For this review, take the finished solid that the model builds, in its own axes (mm). A direction names the side the tool comes from. Round coordinates to 2 decimals unless told otherwise and drop trailing zeros. Write each loop counter-clockwise with the first axis right and the second up, starting at its lowest first coordinate (ties: lowest second). Pieces come first, ordered by that corner, then holes. Notation, with made-up numbers: (85.25, 45.5) - (96.25, 45.5) arc R16 cw to (96.25, 60.5) - close; hole circle Ø10 at (48, -35.75). An arc over 180 degrees is marked (long way). Answer in a Markdown table with one row per item. Add a question column.
from build123d import *

# Parameters (mm, degrees)
SKETCH_2_W               = 20
SKETCH_2_H               = 1.5
SKETCH_2_H_2             = 2.45
CUT_EXTRUDE_1_DEPTH      = 29
CUT_EXTRUDE_1_DEPTH_BACK = 29
CUT_EXTRUDE_2_DEPTH      = 2.45


with BuildPart() as part:
    # Эскиз1 → Повернуть1 (revolve)
    with BuildSketch(Plane.XY):
        Polygon((0, 0), (0, 7), (28, 7), (28, 4), (24.5, 4), (24.5, 2.2), (28, 2.2), (28, 0), align=None)
    revolve(axis=Axis((0, 16.311603896, 0), (0, -1, 0)))

    # Эскиз2 → Вырез-Вытянуть1 (cut, two sides)
    with BuildSketch(Plane.XY) as cut_extrude_1_sk:
        with Locations((18, 6.25)):
            Rectangle(SKETCH_2_W, SKETCH_2_H)
        with Locations((-18, 6.25)):
            Rectangle(SKETCH_2_W, SKETCH_2_H)
        with Locations((18, 1.225)):
            Rectangle(SKETCH_2_W, SKETCH_2_H_2)
        with Locations((-18, 1.225)):
            Rectangle(SKETCH_2_W, SKETCH_2_H_2)
    extrude(amount=CUT_EXTRUDE_1_DEPTH, mode=Mode.SUBTRACT)
    extrude(cut_extrude_1_sk.sketch, amount=-CUT_EXTRUDE_1_DEPTH_BACK, mode=Mode.SUBTRACT)

    # Эскиз3 → Вырез-Вытянуть2 (cut)
    with BuildSketch(Plane.XZ):
        with BuildLine():
            ThreePointArc((8, 26.83281573), (4.850771024, 27.576620904), (1.636756478, 27.952120281))
            Line((1.636756478, 27.952120281), (8, 23.157072354))
            Line((8, 23.157072354), (8, 26.83281573))
        make_face()
        with BuildLine():
            Line((-8, 26.83281573), (-8, 23.157072354))
            Line((-8, 23.157072354), (-1.636756478, 27.952120281))
            ThreePointArc((-1.636756478, 27.952120281), (-4.850771024, 27.576620904), (-8, 26.83281573))
        make_face()
        with BuildLine():
            Line((-1.636756478, -27.952120281), (-8, -23.157072354))
            Line((-8, -23.157072354), (-8, -26.83281573))
            ThreePointArc((-8, -26.83281573), (-4.850771024, -27.576620904), (-1.636756478, -27.952120281))
        make_face()
        with BuildLine():
            Line((8, -23.157072354), (1.636756478, -27.952120281))
            ThreePointArc((1.636756478, -27.952120281), (4.850771024, -27.576620904), (8, -26.83281573))
            Line((8, -26.83281573), (8, -23.157072354))
        make_face()
    extrude(amount=-CUT_EXTRUDE_2_DEPTH, mode=Mode.SUBTRACT)


solid = part.part
Q1. Add section D-D on x = 11.5. State the section outline as (y, z) points.
Q2. Add section C-C on y = 3.25. State the section outline as (x, z) points, then the cut area to 3 significant figures.
Q3. Insertion check: pin 1 Ø2.5 at (y, z) = (1.5, 10) entering from -X; pin 2 Ø4 at (x, z) = (20, -7) entering from -Y; pin 3 Ø1.2 at (y, z) = (6.5, -2) entering from -X. Each pin has a flat end and moves straight along its axis. Give the tip position at first contact, or say it passes through.
Q4. Tool access review of faces 1 (the face through (4.77, 1.08, 25.59)), 2 (the face through (-4.77, 1.08, -25.59)), 3 (the face through (-8, 1, 0)), 4 (the face through (-8, 6, 0)): name each direction out of +Z, -Z, +X, -X, +Y, -Y from which nothing blocks a thin tool from reaching the whole face with its end or side.
Q5. Add section B-B on z = 0. State the section outline as (x, y) points.
Q6. Add section A-A on x = 0. State the section outline as (y, z) points.
Q7. To check wall thickness, follow probe 1 along X at (y, z) = (5.75, 11); probe 2 along X at (y, z) = (3.5, 0); probe 3 along Y at (x, z) = (12.5, 24). State the ranges of each line that lie inside material, in increasing order.
Answer sheet:
| question | item | result |
|---|---|---|
| 1 | outline | (2.45, -21.63) - (4, -21.63) - (4, -25.53) - (5.5, -25.53) - (5.5, 25.53) - (4, 25.53) - (4, 21.63) - (2.45, 21.63) - close |
| 2 | outline | circle Ø49 at (0, 0) |
| 2 | area | 1,890 mm² |
| 3 | pin 1 | stops at x = -22.71 |
| 3 | pin 2 | stops at y = 2.45 |
| 3 | pin 3 | stops at x = -8 |
| 4 | face 1 | +Z, +X, -Y |
| 4 | face 2 | -Z, -X, -Y |
| 4 | face 3 | +Z, -Z, -X, -Y |
| 4 | face 4 | +Z, -Z, -X, +Y |
| 5 | outline | (-28, 4) - (-24.5, 4) - (-24.5, 2.45) - (-8, 2.45) - (-8, 0) - (8, 0) - (8, 2.45) - (24.5, 2.45) - (24.5, 4) - (28, 4) - (28, 5.5) - (8, 5.5) - (8, 7) - (-8, 7) - (-8, 5.5) - (-28, 5.5) - close |
| 6 | outline | (0, -28) - (2.2, -28) - (2.2, -24.5) - (4, -24.5) - (4, -28) - (7, -28) - (7, 28) - (4, 28) - (4, 24.5) - (2.2, 24.5) - (2.2, 28) - (0, 28) - close |
| 7 | probe 1 | x = -8 to 8 |
| 7 | probe 2 | x = -24.5 to 24.5 |
| 7 | probe 3 | y = 4 to 5.5 |
